Here's the drawing with two shaded views (mm, measured from the low corner). I have some questions. Coordinates: 2 decimals unless noted, no trailing zeros. Write each loop counter-clockwise with the first axis right and the second up, starting at its lowest first coordinate (ties: lowest second). Pieces come first, ordered by that corner, then holes. Notation, with made-up numbers: (63.25, 25.5) - (110.25, 25.5) arc R31 cw to (110.25, 61.5) - close; hole circle Ø5 at (-9, 65.25). An arc over 180 degrees is marked (long way). Answer in a Markdown table with one row per item. Add a question column.
Item 1: If I drill on probe 1 along X at (y, z) = (32, 0.2); probe 2 along Y at (x, z) = (67.5, 1.15), over which ranges is the centre line in solid material (lowest first)? Write a range as from..to.
Item 2: Imagine slicing it at B-B (z = 0.5). Please give me the cut outline in (x, y), plus the area to 3 significant figures.
Item 3: I'm going to push flat-ended pins straight in: pin 1 (1 mm diameter, centred on y = 29, z = 0.5, fed in from -X); pin 2 (0.6 mm diameter, centred on y = 1, z = 1, fed in from +X); pin 3 (0.6 mm diameter, centred on x = 72.5, z = 0.5, fed in from +Y); pin 4 (1 mm diameter, centred on y = 1, z = 1, fed in from -X). Where does each tip first touch, or does it pass through?
Item 4: Imagine slicing it at C-C (x = 78.5). Please give me the cut outline in (y, z), plus the area to 3 significant figures.
Item 5: Imagine slicing it at A-A (y = 27.5). Please give me the cut outline in (x, z).
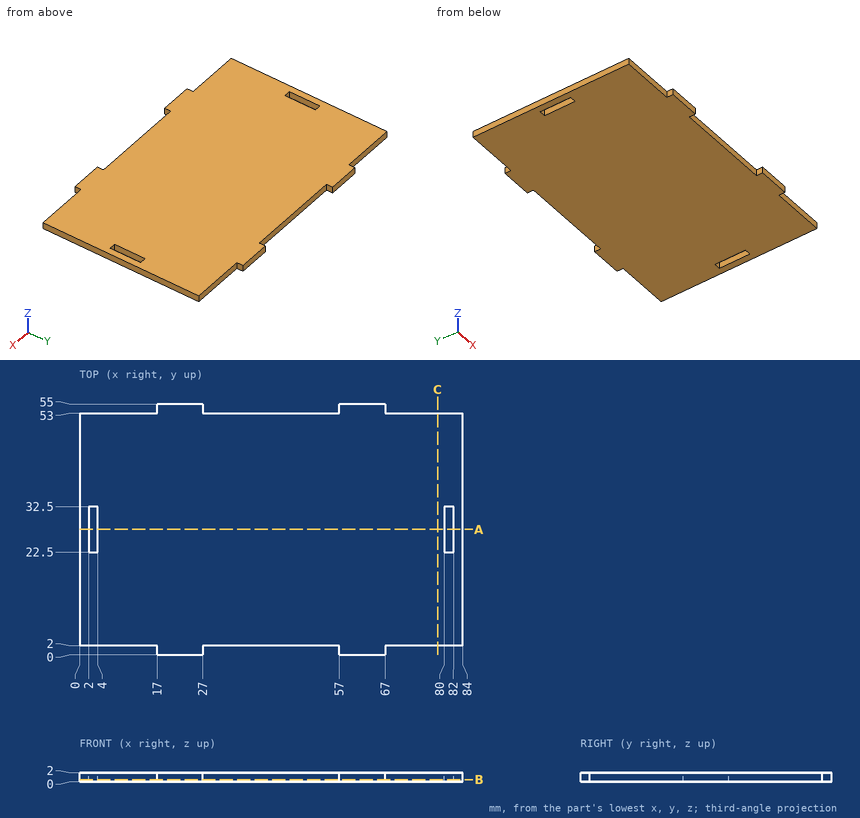
Here are the results:
| question | item | result |
|---|---|---|
| 1 | probe 1 | x = 0..2, 4..80, 82..84 |
| 1 | probe 2 | y = 2..53 |
| 2 | outline | (0, 2) - (17, 2) - (17, 0) - (27, 0) - (27, 2) - (57, 2) - (57, 0) - (67, 0) - (67, 2) - (84, 2) - (84, 53) - (67, 53) - (67, 55) - (57, 55) - (57, 53) - (27, 53) - (27, 55) - (17, 55) - (17, 53) - (0, 53) - close; hole (2, 22.5) - (4, 22.5) - (4, 32.5) - (2, 32.5) - close; hole (80, 22.5) - (82, 22.5) - (82, 32.5) - (80, 32.5) - close |
| 2 | area | 4,320 mm2 |
| 3 | pin 1 | stops at x = 0 |
| 3 | pin 2 | stops at x = 67 |
| 3 | pin 3 | stops at y = 53 |
| 3 | pin 4 | stops at x = 17 |
| 4 | outline | (2, 0) - (53, 0) - (53, 2) - (2, 2) - close |
| 4 | area | 102 mm2 |
| 5 | outline | (0, 0) - (2, 0) - (2, 2) - (0, 2) - close; (4, 0) - (80, 0) - (80, 2) - (4, 2) - close; (82, 0) - (84, 0) - (84, 2) - (82, 2) - close |
